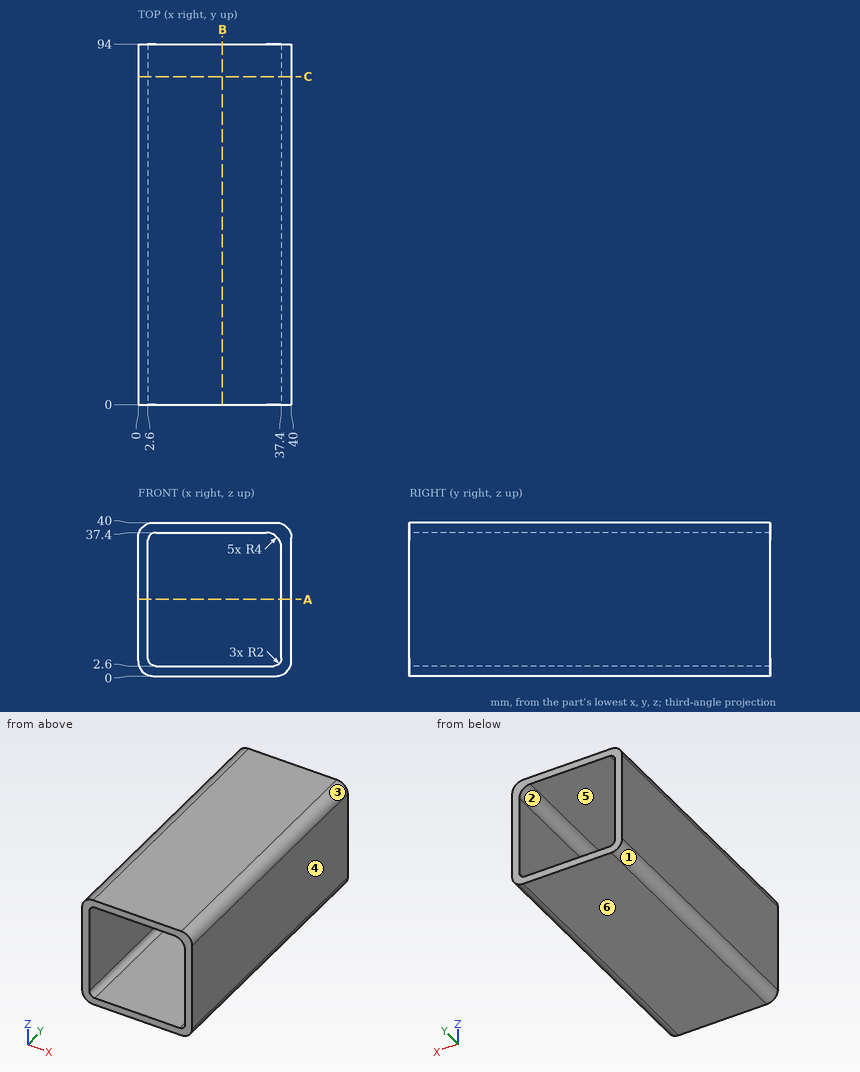
Could you check a few things on this drawing? It's one solid part, dimensions in mm from its lowest x, y, z. A direction names the side the tool comes from. Coordinates: 2 decimals unless noted, no trailing zeros. Order: outer loops, then holes, each group sorted by start corner. A loop starts at its lowest first (then second) coordinate and runs counter-clockwise, first axis right, second up. Notation, with made-up numbers: (-8, 61.25) - (22, 61.25) arc R32 ccw to (22, 92.25) - close; hole circle Ø8 at (-4, 30.5). An arc over 180 degrees is marked (long way). Answer as a JSON object with one key per item and string values. Group by question number.
Q1. On a 3-axis mill with a long thin cutter (end or side, diameter ignored), from which of +Z, -Z, +X, -X, +Y, -Y can I reach the whole of each face in a straight line? I mean the marked faces 5 and 6. Say none if no direction works.
Q2. Will this pin go through, and if not, where does the flat tip stop? P1, Ø12, axis at x = 25, z = 12, coming from the +Y side.
Q3. I need wall thicknesses on line 1 (Z direction, x = 12.5, y = 17.5); line 2 (Z direction, x = 34.5, y = 58.5). Which ranges of each line are inside material? Lowest first, please. Write a range as from..to.
Q4. Imagine slicing it at B-B (x = 22). Please give me the cut outline in (y, z), and give its area (3 significant figures).
Q5. Imagine slicing it at C-C (y = 85.5). Please give me the cut outline in (x, z).
Q6. We'd pull the mould along Z, two halves only. Please class the marked faces 1, 2, 3 and 4: +Z half, -Z half, draft (parallel to the pull), parting line (faces both ways), or undercut.
Q7. Imagine slicing it at A-A (z = 20). Please give me the cut outline in (x, y), and give its area (3 significant figures).
Determined:
{
 "1": {"face 5": "+Y, -Y", "face 6": "-Z, +X, -X, +Y, -Y"},
 "2": {"P1": "passes through"},
 "3": {"line 1": "z = 0..2.6, 37.4..40", "line 2": "z = 0..2.6, 37.25..40"},
 "4": {"outline": "(0, 0) - (94, 0) - (94, 2.6) - (0, 2.6) - close; (0, 37.4) - (94, 37.4) - (94, 40) - (0, 40) - close", "area": "489 mm2"},
 "5": {"outline": "(0, 4) arc R4 ccw to (4, 0) - (36, 0) arc R4 ccw to (40, 4) - (40, 36) arc R4 ccw to (36, 40) - (4, 40) arc R4 ccw to (0, 36) - close; hole (2.6, 4.6) arc R2 ccw to (4.6, 2.6) - (35.4, 2.6) arc R2 ccw to (37.4, 4.6) - (37.4, 33.4) arc R4 ccw to (33.4, 37.4) - (4.6, 37.4) arc R2 ccw to (2.6, 35.4) - close"},
 "6": {"face 1": "-Z half", "face 2": "undercut", "face 3": "+Z half", "face 4": "draft"},
 "7": {"outline": "(0, 0) - (2.6, 0) - (2.6, 94) - (0, 94) - close; (37.4, 0) - (40, 0) - (40, 94) - (37.4, 94) - close", "area": "489 mm2"}
}
